For this review, take the finished solid that the model builds, in its own axes (mm). A direction names the side the tool comes from. Give positions to 0.01 mm unless a question says otherwise; leave off trailing zeros. Order: outer loops, then holes, each group sorted by start corner. A loop starts at its lowest first (then second) coordinate and runs counter-clockwise, first axis right, second up. Notation, with made-up numbers: (-9.5, -5) - (35.5, -5) arc R29 ccw to (35.5, 32) - close; hole circle Ø3 at (-25, 30). An arc over 180 degrees is marked (long way). One line per item, written item: value.
```python
from build123d import *

# Parameters (mm, degrees)
BOSS_EXTRUDE1_DEPTH     = 3
SKETCH2_R               = 2.75
CUT_EXTRUDE1_DEPTH      = 4
SKETCH3_2_R             = 5.75
SKETCH3_2_R_2           = 2.75
BOSS_EXTRUDE3_DEPTH     = 4.5
CUT_EXTRUDE2_DEPTH      = 4.5
BOSS_EXTRUDE4_DEPTH     = 30
CUT_EXTRUDE3_DEPTH      = 57.6
CUT_EXTRUDE3_DEPTH_BACK = 24.4
SKETCH9_R               = 8
SKETCH9_R_2             = 1.75
CUT_EXTRUDE4_DEPTH      = 49.5
CUT_EXTRUDE4_DEPTH_BACK = 52.5
SKETCH3_R               = 5.75
SKETCH3_R_2             = 2.75
BOSS_EXTRUDE2_DEPTH     = 4.5


with BuildPart() as part:
    # Sketch1 → Boss-Extrude1 (new body)
    with BuildSketch(Plane(origin=(0, 0, 0), x_dir=(1, 0, 0), z_dir=(0, 1, 0))):
        with BuildLine():
            Line((-35, 50), (35, 50))
            ThreePointArc((35, 50), (38.535533906, 48.535533906), (40, 45))
            Line((40, 45), (40, -45))
            ThreePointArc((40, -45), (38.535533906, -48.535533906), (35, -50))
            Line((35, -50), (-35, -50))
            ThreePointArc((-35, -50), (-38.535533906, -48.535533906), (-40, -45))
            Line((-40, -45), (-40, 45))
            ThreePointArc((-40, 45), (-38.535533906, 48.535533906), (-35, 50))
        make_face()
    extrude(amount=BOSS_EXTRUDE1_DEPTH)

    # Sketch2 → Cut-Extrude1 (cut, through all)
    with BuildSketch(Plane(origin=(0, 3, 0), x_dir=(1, 0, 0), z_dir=(0, 1, 0))):
        with Locations((-31, 0)):
            Circle(SKETCH2_R)
        with Locations((31, 40)):
            Circle(SKETCH2_R)
        with Locations((31, -40)):
            Circle(SKETCH2_R)
    extrude(amount=-CUT_EXTRUDE1_DEPTH, mode=Mode.SUBTRACT)

    # Sketch3<2> → Boss-Extrude3 (add)
    with BuildSketch(Plane(origin=(0, 3, 0), x_dir=(1, 0, 0), z_dir=(0, 1, 0))):
        with Locations((-31, 0)):
            Circle(SKETCH3_2_R)
        with Locations((-31, 0)):
            Circle(SKETCH3_2_R_2, mode=Mode.SUBTRACT)
        with Locations((31, 40)):
            Circle(SKETCH3_2_R)
        with Locations((31, 40)):
            Circle(SKETCH3_2_R_2, mode=Mode.SUBTRACT)
        with Locations((31, -40)):
            Circle(SKETCH3_2_R)
        with Locations((31, -40)):
            Circle(SKETCH3_2_R_2, mode=Mode.SUBTRACT)
    extrude(amount=BOSS_EXTRUDE3_DEPTH)

    # Sketch6 → Cut-Extrude2 (cut)
    with BuildSketch(Plane(origin=(0, 3, 0), x_dir=(1, 0, 0), z_dir=(0, 1, 0))):
        with BuildLine():
            Line((-36.470429244, -29.778895044), (28.529570756, -49.778895044))
            ThreePointArc((28.529570756, -49.778895044), (29.25652008, -49.944414789), (30, -50))
            Line((30, -50), (-40, -50))
            Line((-40, -50), (-40, -25))
            ThreePointArc((-40, -25), (-39.021948919, -27.970509534), (-36.470429244, -29.778895044))
        make_face()
        with BuildLine():
            Line((-40, 50), (30, 50))
            ThreePointArc((30, 50), (29.25652008, 49.944414789), (28.529570756, 49.778895044))
            Line((28.529570756, 49.778895044), (-36.470429244, 29.778895044))
            ThreePointArc((-36.470429244, 29.778895044), (-39.021948919, 27.970509534), (-40, 25))
            Line((-40, 25), (-40, 50))
        make_face()
    extrude(amount=-CUT_EXTRUDE2_DEPTH, mode=Mode.SUBTRACT)

    # Sketch7 → Boss-Extrude4 (add)
    with BuildSketch(Plane.XZ):
        Polygon((19.6, 6.770211843), (19.6, -6.770211843), (19.6, -31.5), (16.6, -31.5), (16.6, -1.5), (-16.6, -1.5), (-16.6, -31.5), (-19.6, -31.5), (-19.6, -6.770211843), (-19.6, 6.770211843), (-19.6, 31.5), (-16.6, 31.5), (-16.6, 1.5), (16.6, 1.5), (16.6, 31.5), (19.6, 31.5), align=None)
    extrude(amount=BOSS_EXTRUDE4_DEPTH)

    # Sketch8 → Cut-Extrude3 (cut, two sides)
    with BuildSketch(Plane.ZY.offset(-16.6)) as cut_extrude3_sk:
        Polygon((1.5, -30), (31.5, 0), (31.5, -30), align=None)
        Polygon((-1.5, -30), (-31.5, -30), (-31.5, -0.712729134), align=None)
    extrude(amount=CUT_EXTRUDE3_DEPTH, mode=Mode.SUBTRACT)
    extrude(cut_extrude3_sk.sketch, amount=-CUT_EXTRUDE3_DEPTH_BACK, mode=Mode.SUBTRACT)

    # Sketch9 → Cut-Extrude4 (cut, two sides)
    with BuildSketch(Plane(origin=(0, 0, -1.5), x_dir=(-1, 0, 0), z_dir=(0, 0, -1))) as cut_extrude4_sk:
        with Locations((0, -15)):
            Circle(SKETCH9_R)
        with Locations((-8.838834765, -23.838834765)):
            Circle(SKETCH9_R_2)
        with Locations((-8.838834765, -6.161165235)):
            Circle(SKETCH9_R_2)
        with Locations((8.838834765, -23.838834765)):
            Circle(SKETCH9_R_2)
        with Locations((8.838834765, -6.161165235)):
            Circle(SKETCH9_R_2)
    extrude(amount=CUT_EXTRUDE4_DEPTH, mode=Mode.SUBTRACT)
    extrude(cut_extrude4_sk.sketch, amount=-CUT_EXTRUDE4_DEPTH_BACK, mode=Mode.SUBTRACT)

    # Sketch3 → Boss-Extrude2 (add)
    with BuildSketch(Plane(origin=(0, 3, 0), x_dir=(1, 0, 0), z_dir=(0, 1, 0))):
        with Locations((-31, 0)):
            Circle(SKETCH3_R)
        with Locations((-31, 0)):
            Circle(SKETCH3_R_2, mode=Mode.SUBTRACT)
        with Locations((31, 40)):
            Circle(SKETCH3_R)
        with Locations((31, 40)):
            Circle(SKETCH3_R_2, mode=Mode.SUBTRACT)
        with Locations((31, -40)):
            Circle(SKETCH3_R)
        with Locations((31, -40)):
            Circle(SKETCH3_R_2, mode=Mode.SUBTRACT)
    extrude(amount=BOSS_EXTRUDE2_DEPTH)


solid = part.part
```
(1) Draft analysis for pull direction Z (two halves, no side actions). For faces 6 (the face through (29.754, 5.219, 45.613)), 7 (the face through (-39, 2, -28)), 8 (the face through (16.6, -11, 13)), state which applies: pulls with the +Z half, pulls with the -Z half, needs draft (parallel to the pull), parting line crosses it, or undercut.
Answers below:
face 6: undercut
face 7: pulls with the -Z half
face 8: needs draft
(2) Take a section at C-C (z = -40). Write out the cut boundary in (x, y), then the cut area to 3 significant figures.
Answers below:
outline: (-3.25, 0) - (28.25, 0) - (28.25, 7.5) - (25.25, 7.5) - (25.25, 3) - (-3.25, 3) - close; (33.75, 0) - (40, 0) - (40, 3) - (36.75, 3) - (36.75, 7.5) - (33.75, 7.5) - close
area: 140 mm^2
(3) Take a section at B-B (y = -15). Write out the cut boundary in (x, z), then the cut area to 3 significant figures.
Answers below:
outline: (-19.6, -16.87) - (-16.6, -16.87) - (-16.6, -1.5) - (-8, -1.5) - (-8, 1.5) - (-16.6, 1.5) - (-16.6, 16.5) - (-19.6, 16.5) - close; (8, -1.5) - (16.6, -1.5) - (16.6, -16.87) - (19.6, -16.87) - (19.6, 16.5) - (16.6, 16.5) - (16.6, 1.5) - (8, 1.5) - close
area: 252 mm^2
(4) Machinability: for faces 1 (the face through (-39, 2, 28)), 2 (the face through (-16.6, -8, 10)), 3 (the face through (-25.516, 5.219, -1.727)), 4 (the face through (-16.6, -11, -13)), 5 (the face through (-19.6, -11, 0)), which of the approach directions +Z, -Z, +X, -X, +Y, -Y give a long, thin tool a straight path to every point of the face, cutting with its end or side? Answer none if there is none.
Answers below:
face 1: +Z, -X, +Y, -Y
face 2: +Z, -Y
face 3: +Y
face 4: -Z, -Y
face 5: +Z, -Z, -X, -Y
(5) Take a section at A-A (x = -1). Write out the cut boundary in (y, z), then the cut area to 3 significant figures.
Answers below:
outline: (-30, -1.5) - (-22.94, -1.5) - (-22.94, 1.5) - (-30, 1.5) - close; (-7.06, -1.5) - (0, -1.5) - (0, -40.69) - (3, -40.69) - (3, 40.69) - (0, 40.69) - (0, 1.5) - (-7.06, 1.5) - close
area: 287 mm^2
(6) Wall thickness on line 1 (X direction, y = 5, z = 40); line 2 (Y direction, x = 0, z = 0); line 3 (Z direction, x = -31, y = 4): over which ranges is each line inside the solid? List them lowest first. Write a range as from..to.
Answers below:
line 1: x = 25.25..28.25, 33.75..36.75
line 2: y = -30..-23, -7..3
line 3: z = -5.75..-2.75, 2.75..5.75
(7) For P1, Ø9, axis at y = -11.5, z = 16, coming from the +X side; P2, Ø6, axis at x = 0, z = 28, coming from the -Y side; P3, Ø6, axis at x = 25.5, z = 9.5, coming from the +Y side, all flat-tipped, find the tip position at first contact; note any pin that passes through.
Answers below:
P1: stops at x = 19.6
P2: stops at y = 0
P3: stops at y = 3
(8) Take a section at D-D (x = -15). Write out the cut boundary in (y, z), then the cut area to 3 significant figures.
Answers below:
outline: (-30, -1.5) - (0, -1.5) - (0, -36.39) - (3, -36.39) - (3, 36.39) - (0, 36.39) - (0, 1.5) - (-30, 1.5) - close
area: 308 mm^2
